Can you work these out from the model? Positions are in its coordinate system, mm. Round coordinates to 2 decimals unless told otherwise and drop trailing zeros. Order: outer loops, then holes, each group sorted by start corner. A loop starts at its lowest first (then second) coordinate and runs counter-clockwise, first axis right, second up.
from build123d import *

# Parameters (mm, degrees)
SKETCH_1_W          = 10
SKETCH_1_H          = 26
EXTRUDE_1_DEPTH     = 3
SKETCH_2_R          = 1.5
CUT_EXTRUDE_1_DEPTH = 29.017851452


with BuildPart() as part:
    # Эскиз1 → Бобышка-Вытянуть1 (new body)
    with BuildSketch(Plane.XY):
        with Locations((5, 13)):
            Rectangle(SKETCH_1_W, SKETCH_1_H)
    extrude(amount=EXTRUDE_1_DEPTH)

    # Эскиз2 → Вырез-Вытянуть1 (cut, through all)
    with BuildSketch(Plane.XY.offset(3)):
        with Locations((5, 14)):
            Circle(SKETCH_2_R)
    extrude(amount=-CUT_EXTRUDE_1_DEPTH, mode=Mode.SUBTRACT)


solid = part.part
(1) I want a section at A-A, the plane y = 14. List the corners of the cut face in (x, z) for me, plus the area to 3 significant figures.
(2) I want a section at B-B, the plane x = 5. List the corners of the cut face in (y, z) for me.
(3) If we mould it in two halves opening along Y, with no side actions, what happens to faces 1 (the face through (6.386, 13.425, 1.521)), 2 (the face through (10, 13, 1)), 3 (the face through (5, 26, 1)), 4 (the face through (5, 0, 1))? For each: pulls with the +Y half, pulls with the -Y half, needs draft (parallel to the pull), parting line crosses it, or undercut.
(4) I want a section at C-C, the plane z = 1.2. List the corners of the cut face in (x, y) for me.
(5) Please list where these lines run through material, in increasing order: probe 1 along Y at (x, z) = (5, 1.1); probe 2 along Y at (x, z) = (4.5, 0.55).
Ans:
1. outline: (0, 0) - (3.5, 0) - (3.5, 3) - (0, 3) - close; (6.5, 0) - (10, 0) - (10, 3) - (6.5, 3) - close
1. area: 21.0 mm2
2. outline: (0, 0) - (12.5, 0) - (12.5, 3) - (0, 3) - close; (15.5, 0) - (26, 0) - (26, 3) - (15.5, 3) - close
3. face 1: undercut
3. face 2: needs draft
3. face 3: pulls with the +Y half
3. face 4: pulls with the -Y half
4. outline: (0, 0) - (10, 0) - (10, 26) - (0, 26) - close; hole circle Ø3 at (5, 14)
5. probe 1: y = 0 to 12.5, 15.5 to 26
5. probe 2: y = 0 to 12.59, 15.41 to 26
